Check sheet for the modelled part. Datum: model origin and axes. Units: mm. Round coordinates to 2 decimals unless told otherwise and drop trailing zeros. Order: outer loops, then holes, each group sorted by start corner. A loop starts at its lowest first (then second) coordinate and runs counter-clockwise, first axis right, second up. Notation, with made-up numbers: (-17.5, 11.5) -> (23.5, 11.5) arc R23 cw to (23.5, 32.5) -> close; hole circle Ø5 at (-3.75, 89). An arc over 180 degrees is marked (long way). Answer in a Markdown table with one row per item.
from build123d import *

# Parameters (mm, degrees)
F0_W     = 80
F0_H     = 100
F1_DEPTH = 75
F2_R     = 20
F3_DEPTH = 107
F4_R     = 8


with BuildPart() as f1:
    # F0 (on Front) → F1 (new body, symmetric)
    with BuildSketch(Plane.XZ):
        Rectangle(F0_W, F0_H)
    extrude(amount=F1_DEPTH, both=True)

    # F2 (on face) → F3 (cut)
    with BuildSketch(Plane.XY.offset(50)):
        Circle(F2_R)
    extrude(amount=-F3_DEPTH, mode=Mode.SUBTRACT)

    # F4
    f4_edges = [f1.edges().sort_by_distance(p)[0] for p in [
        (40, 0, 50),
        (40, 75, 0),
        (0, 75, 50),
        (-40, 75, 0),
        (0, 75, -50),
        (-40, 0, 50),
        (-40, 0, -50),
        (-40, -75, 0),
        (40, -75, 0),
        (0, -75, 50),
        (0, -75, -50),
        (40, 0, -50),
        (-20, 0, -50),
        (-20, 0, 50),
    ]]
    fillet(f4_edges, radius=F4_R)


solid = f1.part
Item 1: Scan lines: line 1 (Y direction, x = 0, z = 0); line 2 (Y direction, x = -14.5, z = -34); line 3 (Z direction, x = -3, y = -20.5). Record each from-to range of solid material in increasing order. Write a range as [from, to].
Result sheet:
| item | result |
|---|---|
| line 1 | y = [-75, -20], [20, 75] |
| line 2 | y = [-75, -13.77], [13.77, 75] |
| line 3 | z = [-45.31, 45.31] |
Item 2: Cross-section at B-B (z = 27.5). Record the boundary of the cut face in (x, y), and give its area (3 significant figures).
Result sheet:
| item | result |
|---|---|
| outline | (-40, -67) arc R8 ccw to (-32, -75) -> (32, -75) arc R8 ccw to (40, -67) -> (40, 67) arc R8 ccw to (32, 75) -> (-32, 75) arc R8 ccw to (-40, 67) -> close; hole circle Ø40 at (0, 0) |
| area | 10,700 mm^2 |
Item 3: Cross-section at C-C (x = 0). Record the boundary of the cut face in (y, z).
Result sheet:
| item | result |
|---|---|
| outline | (-75, -42) arc R8 ccw to (-67, -50) -> (-28, -50) arc R8 ccw to (-20, -42) -> (-20, 42) arc R8 ccw to (-28, 50) -> (-67, 50) arc R8 ccw to (-75, 42) -> close; (20, -42) arc R8 ccw to (28, -50) -> (67, -50) arc R8 ccw to (75, -42) -> (75, 42) arc R8 ccw to (67, 50) -> (28, 50) arc R8 ccw to (20, 42) -> close |
Item 4: Cross-section at A-A (y = 0). Record the boundary of the cut face in (x, z).
Result sheet:
| item | result |
|---|---|
| outline | (-40, -42) arc R8 ccw to (-32, -50) -> (-28, -50) arc R8 ccw to (-20, -42) -> (-20, 42) arc R8 ccw to (-28, 50) -> (-32, 50) arc R8 ccw to (-40, 42) -> close; (20, -42) arc R8 ccw to (28, -50) -> (32, -50) arc R8 ccw to (40, -42) -> (40, 42) arc R8 ccw to (32, 50) -> (28, 50) arc R8 ccw to (20, 42) -> close |
Item 5: Mould release check, pull along Y, two halves, no side actions. Record for faces 1 (the flat face through (0, -75, 1)), 2 (the cylindrical face through (-37.719, 72.594, 0.588)), 3 (the flat face through (-29, -1, 50)), 4 (the cylindrical face through (-4.336, -19.524, 0.588)): pulls with the +Y half, pulls with the -Y half, needs draft (parallel to the pull), parting line crosses it, or undercut.
Result sheet:
| item | result |
|---|---|
| face 1 | pulls with the -Y half |
| face 2 | pulls with the +Y half |
| face 3 | needs draft |
| face 4 | undercut |
Item 6: Depth check by flat-ended pin: P1, Ø1.5, axis at x = 6, y = -19, coming from the +Z side. Enter the tip coordinate at first touch or a pass-through.
Result sheet:
| item | result |
|---|---|
| P1 | stops at z = 45.22 |
